from build123d import *

# Parameters (mm, degrees)
BOSS_EXTRUDE1_DEPTH   = 0.6
BOSS_EXTRUDE1_2_DEPTH = 0.6
BOSS_EXTRUDE1_3_DEPTH = 0.6
BOSS_EXTRUDE2_DEPTH   = 0.3


with BuildPart() as part:
    # Sketch1 → Boss-Extrude1 (new body)
    with BuildSketch(Plane.XY):
        with BuildLine():
            ThreePointArc((62.865529661, 62.061281034), (48.313215527, 32.007787602), (62.856663932, 1.950002877))
            Line((62.856663932, 1.950002877), (36.497449361, 1.950002877))
            Line((36.497449361, 1.950002877), (23.111234398, 24.145438461))
            Line((23.111234398, 24.145438461), (23.111234398, 1.950002877))
            Line((23.111234398, 1.950002877), (0, 1.950002877))
            Line((0, 1.950002877), (0, 62.061281034))
            Line((0, 62.061281034), (23.3158368, 62.061281034))
            Line((23.3158368, 62.061281034), (36.689087616, 39.887341061))
            Line((36.689087616, 39.887341061), (36.689087616, 62.061281034))
            Line((36.689087616, 62.061281034), (62.865529661, 62.061281034))
        make_face()
    extrude(amount=BOSS_EXTRUDE1_DEPTH)



with BuildPart() as body_2:
    # Sketch1 → Boss-Extrude1 2 (new body)
    with BuildSketch(Plane.XY):
        with BuildLine():
            add(Edge.make_bspline(
                [(55.665817619, 23.934470135), (56.300995164, 21.632545966), (60.312610701, 18.883485306), (68.000137108, 17.687938813), (77.626036713, 18.475223123), (88.050691987, 21.709552098), (99.970855751, 27.901244554), (107.303663525, 33.692026699), (111.490621497, 37.816257369)],
                knots=[0.00273107, 0.00273107, 0.00273107, 0.00273107, 0.111443696, 0.211566761, 0.368518187, 0.562067367, 0.722926062, 1, 1, 1, 1], degree=3))
            Line((111.490621497, 37.816257369), (111.75160581, 36.138246697))
            add(Edge.make_bspline(
                [(61.999805678, 11.574793615), (65.651806063, 11.384741592), (84.022958412, 12.171806498), (105.244079008, 26.24652902), (111.75160581, 36.138246697)],
                knots=[0, 0, 0, 0, 0.285157646, 1, 1, 1, 1], degree=3))
            ThreePointArc((61.999805678, 11.574793615), (115.155551398, 46.516849232), (55.620719661, 24.109610138))
            ThreePointArc((55.620719661, 24.109610138), (55.643144919, 24.022008279), (55.665817619, 23.934470135))
        make_face()
    extrude(amount=BOSS_EXTRUDE1_2_DEPTH)


with BuildPart() as body_3:
    # Sketch1 → Boss-Extrude1 3 (new body)
    with BuildSketch(Plane.XY):
        with BuildLine():
            ThreePointArc((110.412012767, 1.950002877), (124.955461171, 32.007787602), (110.403147038, 62.061281034))
            Line((110.403147038, 62.061281034), (136.46819788, 62.061281034))
            Line((136.46819788, 62.061281034), (136.46819788, 40.00376678))
            Line((136.46819788, 40.00376678), (149.928389856, 62.061281034))
            Line((149.928389856, 62.061281034), (173.268679959, 62.061281034))
            Line((173.268679959, 62.061281034), (136.586879163, 1.950002877))
            Line((136.586879163, 1.950002877), (110.412012767, 1.950002877))
        make_face()
    extrude(amount=BOSS_EXTRUDE1_3_DEPTH)


with BuildPart() as part_1:
    add(part.part)

    add(body_2.part)  # Boss-Extrude2 merges body 2

    add(body_3.part)  # Boss-Extrude2 merges body 3
    # Sketch2 → Boss-Extrude2 (add)
    with BuildSketch(Plane.XY):
        with BuildLine():
            Line((65.288187558, 55.844919694), (56.63383608, 55.844919694))
            ThreePointArc((56.63383608, 55.844919694), (56.398742844, 55.546078646), (56.166626305, 55.244919694))
            Line((56.166626305, 55.244919694), (64.63639539, 55.244919694))
            ThreePointArc((64.63639539, 55.244919694), (64.960215166, 55.547175229), (65.288187558, 55.844919694))
        make_face()
        with BuildLine():
            Line((66.093618581, 7.462059575), (57.201479987, 7.462059575))
            ThreePointArc((57.201479987, 7.462059575), (57.455341197, 7.160746592), (57.7122869, 6.862059575))
            Line((57.7122869, 6.862059575), (66.83249305, 6.862059575))
            ThreePointArc((66.83249305, 6.862059575), (66.460825045, 7.159312475), (66.093618581, 7.462059575))
        make_face()
        with BuildLine():
            Line((54.634511424, 32.386297359), (48.315140731, 32.386297359))
            ThreePointArc((48.315140731, 32.386297359), (48.313307535, 32.086299938), (48.313822955, 31.786297359))
            Line((48.313822955, 31.786297359), (54.632933422, 31.786297359))
            ThreePointArc((54.632933422, 31.786297359), (54.632316231, 32.086301058), (54.634511424, 32.386297359))
        make_face()
        with BuildLine():
            Line((116.067196712, 7.462059575), (107.175058117, 7.462059575))
            ThreePointArc((107.175058117, 7.462059575), (106.807851654, 7.159312475), (106.436183649, 6.862059575))
            Line((106.436183649, 6.862059575), (115.556389799, 6.862059575))
            ThreePointArc((115.556389799, 6.862059575), (115.813335501, 7.160746592), (116.067196712, 7.462059575))
        make_face()
        with BuildLine():
            Line((124.953535967, 32.386297359), (118.634165275, 32.386297359))
            ThreePointArc((118.634165275, 32.386297359), (118.636360468, 32.086301058), (118.635743276, 31.786297359))
            Line((118.635743276, 31.786297359), (124.954853744, 31.786297359))
            ThreePointArc((124.954853744, 31.786297359), (124.955369164, 32.086299938), (124.953535967, 32.386297359))
        make_face()
        with BuildLine():
            Line((116.634840619, 55.844919694), (107.980489141, 55.844919694))
            ThreePointArc((107.980489141, 55.844919694), (108.308461533, 55.547175229), (108.632281309, 55.244919694))
            Line((108.632281309, 55.244919694), (117.102050394, 55.244919694))
            ThreePointArc((117.102050394, 55.244919694), (116.869933855, 55.546078646), (116.634840619, 55.844919694))
        make_face()
    extrude(amount=BOSS_EXTRUDE2_DEPTH)


solid = part_1.part
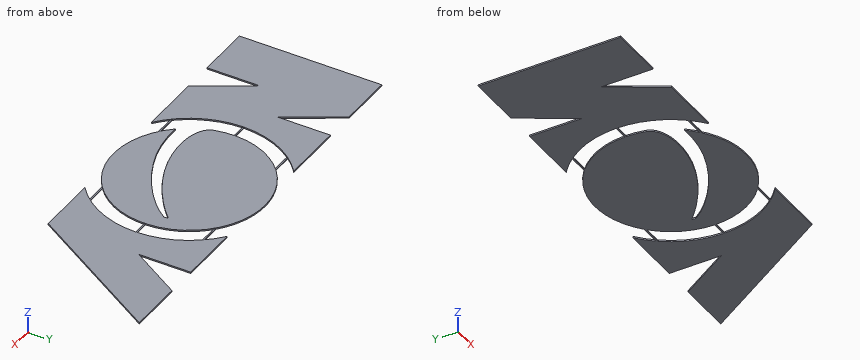
The listing builds one solid part. Answer for the finished solid, in the listing's coordinates (mm). Round coordinates to 2 decimals unless told otherwise and drop trailing zeros. Write each loop counter-clockwise with the first axis right and the second up, starting at its lowest first coordinate (ties: lowest second). Pieces come first, ordered by that corner, then holes. Notation, with made-up numbers: (-6.75, 85.5) - (16.25, 85.5) arc R35 cw to (16.25, 121.5) - close; hole circle Ø2 at (24.5, -11). An arc over 180 degrees is marked (long way). Use a Markdown table: item, result. Add a question column.
1. The part is cut by section C-C (y = 5). Write down the section's boundary in (x, z), and give its area (3 significant figures).
2. The part is cut by section B-B (x = 123). Write down the section's boundary in (y, z).
3. A flat-ended cylindrical pin translates along its axis: P1, Ø1, axis at x = 36, y = 55.5, coming from the +Z side. Find the tip coordinate at first contact, or state that the pin passes through.
4. The part is cut by section A-A (y = 42.5). Write down the section's boundary in (x, z).
5. Consider line 1 (X direction, y = 53, z = 0.15); line 2 (X direction, y = 43, z = 0.45); line 3 (Y direction, x = 61.5, z = 0.35). Determine where each line is inside the solid, lowest interval first.
6. The part is cut by section D-D (x = 20). Write down the section's boundary in (y, z), and give its area (3 significant figures).
Reported:
| question | item | result |
|---|---|---|
| 1 | outline | (0, 0) - (23.11, 0) - (23.11, 0.6) - (0, 0.6) - close; (34.66, 0) - (59.44, 0) - (59.44, 0.6) - (34.66, 0.6) - close; (69.46, 0) - (103.81, 0) - (103.81, 0.6) - (69.46, 0.6) - close; (113.83, 0) - (138.45, 0) - (138.45, 0.6) - (113.83, 0.6) - close |
| 1 | area | 64.1 mm^2 |
| 2 | outline | (1.95, 0) - (19.92, 0) - (19.92, 0.6) - (1.95, 0.6) - close; (31.79, 0) - (32.39, 0) - (32.39, 0.3) - (31.79, 0.3) - close; (44.09, 0) - (62.06, 0) - (62.06, 0.6) - (44.09, 0.6) - close |
| 3 | P1 | through |
| 4 | outline | (0, 0) - (35.11, 0) - (35.11, 0.6) - (0, 0.6) - close; (36.69, 0) - (49.78, 0) - (49.78, 0.6) - (36.69, 0.6) - close; (56.4, 0) - (116.87, 0) - (116.87, 0.6) - (56.4, 0.6) - close; (123.49, 0) - (136.47, 0) - (136.47, 0.6) - (123.49, 0.6) - close; (137.99, 0) - (161.33, 0) - (161.33, 0.6) - (137.99, 0.6) - close |
| 5 | line 1 | 0 to 28.78, 36.69 to 54.58, 62.48 to 110.78, 118.69 to 136.47, 144.4 to 167.74 |
| 5 | line 2 | 0 to 34.81, 36.69 to 49.93, 56.58 to 116.69, 123.34 to 136.47, 138.3 to 161.64 |
| 5 | line 3 | 1.95 to 3.08, 19 to 51.81, 60.93 to 62.06 |
| 6 | outline | (1.95, 0) - (62.06, 0) - (62.06, 0.6) - (1.95, 0.6) - close |
| 6 | area | 36.1 mm^2 |
